Work out the finished part from the listing and answer in its coordinate system (mm). A direction names the side the tool comes from. Coordinates: 2 decimals unless noted, no trailing zeros. Write each question's results on one line, items separated by ' | '.
```python
from build123d import *

# Parameters (mm, degrees)
F3_DEPTH = 3.175


with BuildPart() as f1:
    # F0 (on Front) → F1 (revolve)
    with BuildSketch(Plane.XZ):
        with BuildLine():
            ThreePointArc((-12.7, 336.55), (-10.840128, 332.059872), (-6.35, 330.2))
            Line((-6.35, 330.2), (6.35, 330.2))
            ThreePointArc((6.35, 330.2), (10.840128, 332.059872), (12.7, 336.55))
            Line((12.7, 336.55), (12.7, 355.6))
            ThreePointArc((12.7, 355.6), (8.980256, 364.580256), (0, 368.3))
            ThreePointArc((0, 368.3), (-8.980256, 364.580256), (-12.7, 355.6))
            Line((-12.7, 355.6), (-12.7, 336.55))
        make_face()
    revolve(axis=Axis((-90.849288, 0, 0), (-1, 0, 0)))

    # F2 (on Right) → F3 (join, symmetric)
    with BuildSketch(Plane.YZ):
        Polygon((-12.7, 0), (0, 0), (0, 330.2), (-25.4, 330.2), align=None)
    extrude(amount=F3_DEPTH, both=True)


solid = f1.part
```
1) Straight lines are drawn through the part: probe 1 along Y at (x, z) = (-2, 189); probe 2 along Z at (x, y) = (4, -260); probe 3 along Y at (x, z) = (0.5, -27). For each, find the intervals that lie inside material, in ascending order. Write a range as [from, to].
Check result:
probe 1: [-315.92, -270.76], [-19.97, 0], [270.76, 315.92] | probe 2: [-259.94, -203.55], [203.55, 259.94] | probe 3: [-367.3, -329.09], [329.09, 367.3]
2) Find section A-A, the plane z = 99. Give the number of separate pieces and of enclosed holes in the cut face, and give its area (3 significant figures).
Check result:
separate pieces: 3 | enclosed holes: 0 | area: 1,940 mm^2
3) Given pin 1 Ø7.5 at (y, z) = (-12, 130) entering from -X (3 decimals); pin 2 Ø7 at (x, z) = (1.5, 243) entering from +Y; pin 3 Ø10 at (x, y) = (-1, -230.5) entering from +Z, each flat-ended and moving along its own axis, determine where each tip first touches the part or whether it passes through.
Check result:
pin 1: x = -3.175 | pin 2: y = 279.71 | pin 3: z = 291.16
4) Which of the six approach directions +Z, -Z, +X, -X, +Y, -Y give full straight-line access (tool end or side, diameter ignored) to faces 3 (the face through (12.7, 212, -262)), 4 (the face through (3.175, -10, 167))?
Check result:
face 3: +Z, -Z, +X, +Y, -Y | face 4: +X
5) For a pull along Z with two mould halves and no side action, classify faces 1 (the face through (-12.7, 212, 262)), 2 (the face through (-3.175, -10, 167)) as released by +Z, released by -Z, zero draft, split by the parting line, or undercut.
Check result:
face 1: zero draft | face 2: undercut
